```python
from build123d import *

# Parameters (mm, degrees)
F0_W     = 38.1
F0_H     = 38.1
F1_DEPTH = 330.2
F2_R     = 12.7
F3_DEPTH = 38.101
F4_R     = 12.7


with BuildPart() as f1:
    # F0 (on Front) → F1 (new body)
    with BuildSketch(Plane.XZ):
        with Locations((-3.677602, 3.30648)):
            Rectangle(F0_W, F0_H)
    extrude(amount=F1_DEPTH)

    # F2 (on face) → F3 (cut, through all)
    with BuildSketch(Plane.YZ.offset(15.372398)):
        with Locations((-303.540766, 3.30648)):
            Circle(F2_R)
    extrude(amount=-F3_DEPTH, mode=Mode.SUBTRACT)

    # F4
    f4_edges = [f1.edges().sort_by_distance(p)[0] for p in [
        (-3.677602, -330.2, 22.35648),
        (-3.677602, -330.2, -15.74352),
    ]]
    fillet(f4_edges, radius=F4_R)


solid = f1.part
```
Geometry: final body of the model. Coordinates: model frame, mm. Round coordinates to 2 decimals unless told otherwise and drop trailing zeros. Write each loop counter-clockwise with the first axis right and the second up, starting at its lowest first coordinate (ties: lowest second). Pieces come first, ordered by that corner, then holes. Notation, with made-up numbers: M 61.25,-11 L 70.25,-11 A10 cw 70.25,5 Z; hole C -20.75,54.5 d7. An arc over 180 degrees is marked long. Answer in a Markdown table with one row per item. Add a question column.
(1) Ray query, L1, parallel to Y at x = 4.5, z = 10; L2, parallel to Y at x = -3, z = 1.5; L3, parallel to Y at x = 0, z = -12. Return the intervals inside material, ascending.
(2) Cut plane B-B, the plane x = 3.5. Return the cut outline in (y, z), then the cut area to 3 significant figures.
(3) Cut plane A-A, the plane z = 6. Return the cut outline in (x, y).
(4) Contact query for a flat-ended pin moving along its axis: pin 1 (2 mm diameter, centred on x = -12.5, z = 16.5, fed in from -Y). Output: stop coordinate, or through.
(5) Draft query along Y for faces 1 (the face through (-3.41, -316.23, 3.86)), 2 (the face through (-4, -157, 22.356)), 3 (the face through (-3.411, -326.578, 18.537)). Return one class per face: pulls with the +Y half, pulls with the -Y half, needs draft (parallel to the pull), parting line crosses it, or undercut.
Established:
| question | item | result |
|---|---|---|
| 1 | L1 | -330.2 to -314.33, -292.75 to 0 |
| 1 | L2 | -330.2 to -316.11, -290.97 to 0 |
| 1 | L3 | -326.5 to 0 |
| 2 | outline | M -330.2,-3.04 A12.7 ccw -317.5,-15.74 L 0,-15.74 L 0,22.36 L -317.5,22.36 A12.7 ccw -330.2,9.66 Z; hole C -303.54,3.31 d25.4 |
| 2 | area | 12,000 mm² |
| 3 | outline | M -22.73,-330.2 L 15.37,-330.2 L 15.37,-315.95 L -22.73,-315.95 Z; M -22.73,-291.13 L 15.37,-291.13 L 15.37,0 L -22.73,0 Z |
| 4 | pin 1 | y = -328.78 |
| 5 | face 1 | undercut |
| 5 | face 2 | needs draft |
| 5 | face 3 | pulls with the -Y half |
